Check sheet for the modelled part. Datum: model origin and axes. Units: mm. Coordinates: 2 decimals unless noted, no trailing zeros. Write each loop counter-clockwise with the first axis right and the second up, starting at its lowest first coordinate (ties: lowest second). Pieces come first, ordered by that corner, then holes. Notation, with made-up numbers: (47.25, 52.25) - (59.25, 52.25) arc R22 ccw to (59.25, 80.25) - close; hole circle Ø6 at (84.5, 57). An arc over 180 degrees is marked (long way). Use one line per item in the form item = value. Start each with the question number.
1. Cross-section at B-B on x = 16.5. Record the boundary of the cut face in (y, z) (3 decimals), then the cut area to 3 significant figures.
2. Scan lines: line 1 along X through (y, z) = (1.65, -21.5); line 2 along Z through (x, y) = (67, 2.7) (3 decimals); line 3 along Z through (x, y) = (63, 1.85). Record each from-to range of solid material in increasing order.
3. Cross-section at C-C on z = -48.5. Record the boundary of the cut face in (x, y) (3 decimals), then the cut area to 3 significant figures.
4. Cross-section at D-D on y = 0.5. Give the number of separate pieces and of enclosed holes in the cut face, then the cut area to 3 significant figures.
5. Go/stop test with flat-tipped pins: pin 1 Ø1 at (x, y) = (79.5, 1.5) entering from +Z; pin 2 Ø1.6 at (y, z) = (1, -71.5) entering from +X; pin 3 Ø1 at (y, z) = (1, -72) entering from -X. Record where each tip stops, or that it passes through.
6. Cross-section at A-A on z = -21.5. Record the boundary of the cut face in (x, y) (3 decimals).
```python
from build123d import *

# Parameters (mm, degrees)
SKETCH1_W                 = 100
SKETCH1_H                 = 70
BOSS_EXTRUDE1_DEPTH       = 3.175
SKETCH3_W                 = 3.175
SKETCH3_H                 = 10
SKETCH3_W_2               = 10
SKETCH3_H_2               = 3.175
BOSS_EXTRUDE2_DEPTH       = 3.175
MIRROR2_COPY_1_SKETCH_W   = 3.175
MIRROR2_COPY_1_SKETCH_H   = 10
MIRROR2_COPY_1_SKETCH_W_2 = 10
MIRROR2_COPY_1_SKETCH_H_2 = 3.175
MIRROR2_COPY_1_DEPTH      = 3.175
MIRROR2_COPY_2_SKETCH_W   = 3.175
MIRROR2_COPY_2_SKETCH_H   = 10
MIRROR2_COPY_2_SKETCH_W_2 = 10
MIRROR2_COPY_2_SKETCH_H_2 = 3.175
MIRROR2_COPY_2_DEPTH      = 3.175
CUT_EXTRUDE1_DEPTH        = 127.529608689
CUT_EXTRUDE1_DEPTH_BACK   = 127.529608689
SKETCH4_W                 = 20
SKETCH4_H                 = 32
SKETCH4_W_2               = 7
SKETCH4_H_2               = 7
SKETCH4_W_3               = 15
SKETCH4_H_3               = 15
FILLET1_R                 = 2
CUT_EXTRUDE2_DEPTH        = 127.529608689
CUT_EXTRUDE2_DEPTH_BACK   = 127.529608689
SKETCH5_R                 = 10


with BuildPart() as part:
    # Sketch1 → Boss-Extrude1 (new body)
    with BuildSketch(Plane(origin=(0, 0, 0), x_dir=(1, 0, 0), z_dir=(0, 1, 0))):
        with Locations((50, 35)):
            Rectangle(SKETCH1_W, SKETCH1_H)
    extrude(amount=BOSS_EXTRUDE1_DEPTH)

    # Sketch3 → Boss-Extrude2 (add)
    with BuildSketch(Plane(origin=(0, 0, 0), x_dir=(1, 0, 0), z_dir=(0, 1, 0))):
        with Locations((-1.5875, 55)):
            Rectangle(SKETCH3_W, SKETCH3_H)
        with Locations((-1.5875, 35)):
            Rectangle(SKETCH3_W, SKETCH3_H)
        with Locations((-1.5875, 15)):
            Rectangle(SKETCH3_W, SKETCH3_H)
        with Locations((30, 71.5875)):
            Rectangle(SKETCH3_W_2, SKETCH3_H_2)
        with Locations((70, 71.5875)):
            Rectangle(SKETCH3_W_2, SKETCH3_H_2)
        with Locations((90, 71.5875)):
            Rectangle(SKETCH3_W_2, SKETCH3_H_2)
        with Locations((10, 71.5875)):
            Rectangle(SKETCH3_W_2, SKETCH3_H_2)
        with Locations((50, 71.5875)):
            Rectangle(SKETCH3_W_2, SKETCH3_H_2)
    boss_extrude2 = extrude(amount=BOSS_EXTRUDE2_DEPTH)

    # Mirror1: Boss-Extrude2 across plane
    add(boss_extrude2.mirror(Plane(origin=(50, 0, 0), x_dir=(0, 0, 1), z_dir=(1, 0, 0))))

    # Mirror2 copy 1 sketch → Mirror2 copy 1 (add)
    with BuildSketch(Plane(origin=(100, 0, -70), x_dir=(-1, 0, 0), z_dir=(0, 1, 0))):
        with Locations((-1.5875, 55)):
            Rectangle(MIRROR2_COPY_1_SKETCH_W, MIRROR2_COPY_1_SKETCH_H)
        with Locations((-1.5875, 35)):
            Rectangle(MIRROR2_COPY_1_SKETCH_W, MIRROR2_COPY_1_SKETCH_H)
        with Locations((-1.5875, 15)):
            Rectangle(MIRROR2_COPY_1_SKETCH_W, MIRROR2_COPY_1_SKETCH_H)
        with Locations((30, 71.5875)):
            Rectangle(MIRROR2_COPY_1_SKETCH_W_2, MIRROR2_COPY_1_SKETCH_H_2)
        with Locations((70, 71.5875)):
            Rectangle(MIRROR2_COPY_1_SKETCH_W_2, MIRROR2_COPY_1_SKETCH_H_2)
        with Locations((90, 71.5875)):
            Rectangle(MIRROR2_COPY_1_SKETCH_W_2, MIRROR2_COPY_1_SKETCH_H_2)
        with Locations((10, 71.5875)):
            Rectangle(MIRROR2_COPY_1_SKETCH_W_2, MIRROR2_COPY_1_SKETCH_H_2)
        with Locations((50, 71.5875)):
            Rectangle(MIRROR2_COPY_1_SKETCH_W_2, MIRROR2_COPY_1_SKETCH_H_2)
    extrude(amount=MIRROR2_COPY_1_DEPTH)

    # Mirror2 copy 2 sketch → Mirror2 copy 2 (add)
    with BuildSketch(Plane(origin=(0, 0, -70), x_dir=(1, 0, 0), z_dir=(0, 1, 0))):
        with Locations((-1.5875, -55)):
            Rectangle(MIRROR2_COPY_2_SKETCH_W, MIRROR2_COPY_2_SKETCH_H)
        with Locations((-1.5875, -35)):
            Rectangle(MIRROR2_COPY_2_SKETCH_W, MIRROR2_COPY_2_SKETCH_H)
        with Locations((-1.5875, -15)):
            Rectangle(MIRROR2_COPY_2_SKETCH_W, MIRROR2_COPY_2_SKETCH_H)
        with Locations((30, -71.5875)):
            Rectangle(MIRROR2_COPY_2_SKETCH_W_2, MIRROR2_COPY_2_SKETCH_H_2)
        with Locations((70, -71.5875)):
            Rectangle(MIRROR2_COPY_2_SKETCH_W_2, MIRROR2_COPY_2_SKETCH_H_2)
        with Locations((90, -71.5875)):
            Rectangle(MIRROR2_COPY_2_SKETCH_W_2, MIRROR2_COPY_2_SKETCH_H_2)
        with Locations((10, -71.5875)):
            Rectangle(MIRROR2_COPY_2_SKETCH_W_2, MIRROR2_COPY_2_SKETCH_H_2)
        with Locations((50, -71.5875)):
            Rectangle(MIRROR2_COPY_2_SKETCH_W_2, MIRROR2_COPY_2_SKETCH_H_2)
    extrude(amount=MIRROR2_COPY_2_DEPTH)

    # Sketch4 → Cut-Extrude1 (cut, two sides: drawn at the far end of the back side and taken through both)
    with BuildSketch(Plane.XZ.offset(-CUT_EXTRUDE1_DEPTH_BACK)):
        with Locations((60, -26)):
            Rectangle(SKETCH4_W, SKETCH4_H)
        with Locations((60, -55.5)):
            Rectangle(SKETCH4_W_2, SKETCH4_H_2)
        with Locations((85, -35)):
            Rectangle(SKETCH4_W_3, SKETCH4_H_3)
    extrude(amount=CUT_EXTRUDE1_DEPTH + CUT_EXTRUDE1_DEPTH_BACK, mode=Mode.SUBTRACT)

    # Fillet1
    fillet1_edges = [part.edges().sort_by_distance(p)[0] for p in [
        (77.5, 1.5875, -42.5),
        (77.5, 1.5875, -27.5),
        (92.5, 1.5875, -27.5),
        (92.5, 1.5875, -42.5),
    ]]
    fillet(fillet1_edges, radius=FILLET1_R)

    # Sketch5 → Cut-Extrude2 (cut, two sides: drawn at the far end of the back side and taken through both)
    with BuildSketch(Plane.XZ.offset(-CUT_EXTRUDE2_DEPTH_BACK)):
        with Locations(Location((25, -48.5, 0), (0, 0, 270))):
            Circle(SKETCH5_R)
        with Locations(Location((25, -21.5, 0), (0, 0, 270))):
            Circle(SKETCH5_R)
    extrude(amount=CUT_EXTRUDE2_DEPTH + CUT_EXTRUDE2_DEPTH_BACK, mode=Mode.SUBTRACT)


solid = part.part
```
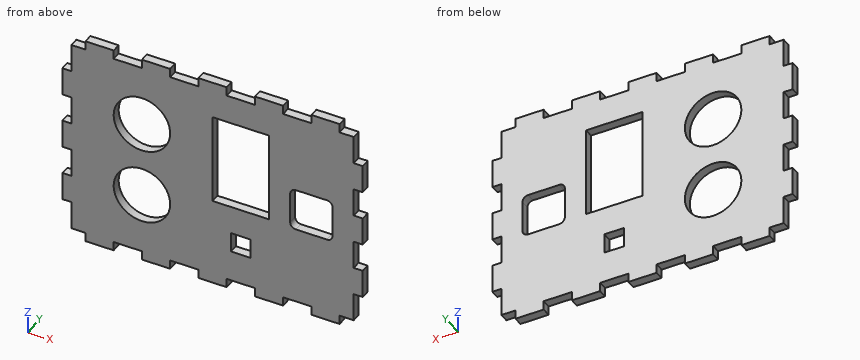
Final values:
q1.outline = (0, -70) - (3.175, -70) - (3.175, -53.768) - (0, -53.768) - close; (0, -43.232) - (3.175, -43.232) - (3.175, -26.768) - (0, -26.768) - close; (0, -16.232) - (3.175, -16.232) - (3.175, 0) - (0, 0) - close
q1.area = 155 mm²
q2.line_1 = 0 to 15, 35 to 50, 70 to 100
q2.line_2 = -73.175 to -42, -10 to 3.175
q2.line_3 = -70 to -59, -52 to -42, -10 to 0
q3.outline = (0, 0) - (15, 0) - (15, 3.175) - (0, 3.175) - close; (35, 0) - (100, 0) - (100, 3.175) - (35, 3.175) - close
q3.area = 254 mm²
q4.separate_pieces = 1
q4.enclosed_holes = 5
q4.area = 5,970 mm²
q5.pin_1 = 0
q5.pin_2 = 95
q5.pin_3 = 5
q6.outline = (0, 0) - (15, 0) - (15, 3.175) - (0, 3.175) - close; (35, 0) - (50, 0) - (50, 3.175) - (35, 3.175) - close; (70, 0) - (100, 0) - (100, 3.175) - (70, 3.175) - close
